Geometry: final body of the model. Coordinates: model frame, mm. Give positions to 0.01 mm unless a question says otherwise; leave off trailing zeros. Write each loop counter-clockwise with the first axis right and the second up, starting at its lowest first coordinate (ties: lowest second). Pieces come first, ordered by that corner, then holes. Notation, with made-up numbers: (-25.75, -36) -> (-12.75, -36) arc R19 ccw to (-12.75, -9) -> close; hole circle Ø2 at (-6, -21.5). An arc over 180 degrees is marked (long way). Answer as a JSON object with one key per item and string values.
Autodesk Inventor part; units mm, degrees
ref_plane "YZ Plane" through (0, 0, 0) normal (1, 0, 0) x (0, 1, 0)
ref_plane "XZ Plane" through (0, 0, 0) normal (0, 1, 0) x (-1, 0, 0)
sketch "Sketch1" plane through (0, 0, 0) normal (0, 0, 1) x (1, 0, 0)
  line L0 (0, 10) -> (-14.2265, 10)
  line L1 (-14.2265, 10) -> (-138.453, 225.1666)
  line L2 (-138.453, 225.1666) -> (-150, 225.1666)
  line L3 (-150, 225.1666) -> (-20, 0)
  line L4 (-20, 0) -> (0, 0)
  line L5 (0, 0) -> (0, 10)
  dimension "d0" = 260
  dimension "d1" = 30
  dimension "d2" = 10
  dimension "d3" = 10
  dimension "d4" = 20
extrude "Extrusion1" add sketch "Sketch1" along normal mid plane 5
mirror "Mirror1" about plane through (0, 0, 0) normal (1, 0, 0) of "Extrusion1"
ref_plane "Work Plane1" through (138.453, 225.1666, 2.5) normal (0, -1, 0) x (0, 0, -1)
sketch "Sketch2" plane through (138.453, 225.1666, 2.5) normal (0, -1, 0) x (0, 0, -1)
  line L0 (2.5, -348.453) -> (2.5, 71.547) construction
  line L1 (5, 0) -> (0, 0) construction
  line L2 (5, 11.547) -> (0, 11.547) construction
  line L3 (0, 0) -> (0, 11.547) construction
  line L4 (5, 11.547) -> (5, 0) construction
  line L5 (2.5, 11.547) -> (2.5, 0) construction
  line L6 (5, -276.906) -> (0, -276.906) construction
  line L7 (0, -276.906) -> (0, -288.453) construction
  line L8 (5, -288.453) -> (0, -288.453) construction
  line L9 (5, -288.453) -> (5, -276.906) construction
  line L10 (2.5, -276.906) -> (2.5, -288.453) construction
  line L11 (2.5, 5.7735) -> (2.5, -282.6795)
  line L12 (0, -288.453) -> (0, -158.453) construction
  point P0 (2.5, -138.453)
sketch "Sketch3" plane through (-20, 0, -2.5) normal (0, -1, 0) x (1, 0, 0)
  point P0 (20, 2.5)
  point P1 (20, 2.5)
properties part number "Braccetto"
Q1. Mould query, pull axis X, two halves, no side actions, for faces 1 (the flat face through (77.21, 119.09, -0.04)), 2 (the flat face through (55, 80, 2.5)), 3 (the flat face through (84.09, 111.01, -0.04)), 4 (the flat face through (-75.47, 116.08, -0.04)). Classes: pulls with the +X half, pulls with the -X half, needs draft (parallel to the pull), parting line crosses it, or undercut.
Values:
{"face 1": "undercut", "face 2": "needs draft", "face 3": "pulls with the +X half", "face 4": "undercut"}
Q2. Cut plane B-B (y = 145). Return the cut outline in (x, z), and give its area (3 significant figures).
Values:
{"outline": "(-103.72, -2.5) -> (-92.17, -2.5) -> (-92.17, 2.5) -> (-103.72, 2.5) -> close; (92.17, -2.5) -> (103.72, -2.5) -> (103.72, 2.5) -> (92.17, 2.5) -> close", "area": "115 mm²"}
Q3. Material intervals for L1, parallel to X at y = 159, z = -0.7; L2, parallel to X at y = 134, z = 0.9; L3, parallel to Y at x = -68, z = -0.95, sorted ascending. Write a range as from..to.
Values:
{"L1": "-111.8..-100.25, 100.25..111.8", "L2": "-97.36..-85.82, 85.82..97.36", "L3": "83.14..103.14"}
Q4. Cut plane C-C (x = 43). Return the cut outline in (y, z).
Values:
{"outline": "(39.84, -2.5) -> (59.84, -2.5) -> (59.84, 2.5) -> (39.84, 2.5) -> close"}
Q5. Cut plane A-A (z = 1.55). Return the cut outline in (x, y), and give its area (3 significant figures).
Values:
{"outline": "(-150, 225.17) -> (-20, 0) -> (20, 0) -> (150, 225.17) -> (138.45, 225.17) -> (14.23, 10) -> (-14.23, 10) -> (-138.45, 225.17) -> close", "area": "5,430 mm²"}
Q6. First-contact query: P1, Ø2, axis at x = 119.5, z = 1.5, coming from the -Y side; P2, Ø1, axis at x = 64.5, z = -0.5, coming from the -Y side; P3, Ø1.5, axis at y = 24, z = -1, coming from the +X side. Flat tips, straight axial feed; report the tip coordinate or a pass-through.
Values:
{"P1": "y = 170.61", "P2": "y = 76.21", "P3": "x = 34.29"}
